Design review of the part built by this model. Coordinates are the model's own, in mm. A direction names the side the tool comes from. Coordinates: 2 decimals unless noted, no trailing zeros. Loops run counter-clockwise (first coordinate to the right, second up) from the corner with the lowest first, then second, coordinate; pieces in that order, holes last.
Q1. For P1, Ø0.6, axis at y = 4.5, z = 0.5, coming from the +X side; P2, Ø0.6, axis at x = -17, z = 1, coming from the -Y side, all flat-tipped, find the tip position at first contact; note any pin that passes through.
Q2. Draft analysis for pull direction Y (two halves, no side actions). For faces 6 (the face through (0.3, 10.305, -0.5)), 7 (the face through (0.252, 4.38, 0.914)), 8 (the face through (0, 14, -1.024)), state which applies: released by +Y, released by -Y, zero draft, split by the parting line, or undercut.
Q3. Add section C-C on y = 4.25. Give the boundary of the cut face in (x, z), and give its area (3 significant figures).
Q4. Machinability: for faces 1 (the face through (0, 8, -0.024)), 2 (the face through (-16, 4, 0.4)), 3 (the face through (16, 4, 0.4)), 4 (the face through (-18, 13, 0)), 5 (the face through (-17.715, 18.003, 0.256)), which of the approach directions +Z, -Z, +X, -X, +Y, -Y give a long, thin tool a straight path to every point of the face, cutting with its end or side? Answer none if there is none.
Q5. Add section A-A on x = 0. Give the boundary of the cut face in (y, z), and give its area (3 significant figures).
Q6. Wall thickness on probe 1 along Y at (x, z) = (-13, -0.55); probe 2 along Z at (x, y) = (-8, 7.25); probe 3 along Z at (x, y) = (-5, 4.5): over which ranges is each line inside the solid? List them lowest first.
Q7. Add section B-B on y = 8.25. Give the boundary of the cut face in (x, z).
```python
from build123d import *

# Parameters (mm, degrees)
BOSS_EXTRUDE1_DEPTH      = 1.5
BOSS_EXTRUDE1_DEPTH_BACK = 1.2
CUT_EXTRUDE1_DEPTH       = 40


with BuildPart() as part:
    # Sketch1 → Boss-Extrude1 (new body, two sides)
    with BuildSketch(Plane.XY) as boss_extrude1_sk:
        with BuildLine():
            Line((-17.999999991, 9.304537824), (-17.999999991, 10.304506021))
            Line((-17.999999991, 10.304506021), (-17.999999991, 17.303464443))
            ThreePointArc((-17.999999991, 17.303464443), (-17.707106772, 18.010571225), (-16.999999991, 18.303464443))
            Line((-16.999999991, 18.303464443), (16.999968161, 18.303464443))
            ThreePointArc((16.999968161, 18.303464443), (17.707074942, 18.010571225), (17.999968161, 17.303464443))
            Line((17.999968161, 17.303464443), (17.999968161, 9.303464443))
            Line((17.999968161, 9.303464443), (17.999968161, 6.751174458))
            ThreePointArc((17.999968161, 6.751174458), (17.707074942, 6.044067677), (16.999968161, 5.751174458))
            Line((16.999968161, 5.751174458), (16.499999991, 5.751174458))
            ThreePointArc((16.499999991, 5.751174458), (16.1464466, 5.604727849), (15.999999991, 5.251174458))
            Line((15.999999991, 5.251174458), (15.999999991, 2.751174458))
            ThreePointArc((15.999999991, 2.751174458), (15.707106772, 2.044067677), (14.999999991, 1.751174458))
            Line((14.999999991, 1.751174458), (-14.999999991, 1.751174458))
            ThreePointArc((-14.999999991, 1.751174458), (-15.707106772, 2.044067677), (-15.999999991, 2.751174458))
            Line((-15.999999991, 2.751174458), (-15.999999991, 5.251174458))
            ThreePointArc((-15.999999991, 5.251174458), (-16.1464466, 5.604727849), (-16.499999991, 5.751174458))
            Line((-16.499999991, 5.751174458), (-16.999999991, 5.751174458))
            ThreePointArc((-16.999999991, 5.751174458), (-17.707106772, 6.044067677), (-17.999999991, 6.751174458))
            Line((-17.999999991, 6.751174458), (-17.999999991, 9.304537824))
        make_face()
    extrude(amount=BOSS_EXTRUDE1_DEPTH)
    extrude(boss_extrude1_sk.sketch, amount=-BOSS_EXTRUDE1_DEPTH_BACK)

    # Sketch3 → Cut-Extrude1 (cut)
    with BuildSketch(Plane(origin=(17.999968161, 0, 0), x_dir=(0, 0, -1), z_dir=(1, 0, 0))):
        with BuildLine():
            Line((0.023796664, 6.751174458), (0.023796664, 5.754537824))
            ThreePointArc((0.023796664, 5.754537824), (0.053060483, 3.748723952), (0.23729316, 1.751174458))
            Line((0.23729316, 1.751174458), (1.2708887, 1.751174458))
            Line((1.2708887, 1.751174458), (1.2708887, 10.304537824))
            Line((1.2708887, 10.304537824), (1.2708887, 10.30507849))
            ThreePointArc((1.2708887, 10.30507849), (7.212872074, 16.614024598), (1.023796664, 22.680762846))
            Line((1.023796664, 22.680762846), (1.023796664, 17.303464443))
            Line((1.023796664, 17.303464443), (1.2, 17.303464443))
            Line((1.2, 17.303464443), (1.2, 6.751174458))
            Line((1.2, 6.751174458), (0.023796664, 6.751174458))
        make_face()
        Polygon((0.023796664, 10.304537824), (0.023796664, 6.751174458), (1.2, 6.751174458), (1.2, 17.303464443), (1.023796664, 17.303464443), (1.023796664, 10.304537824), align=None)
        with BuildLine():
            ThreePointArc((-1.485404738, 6.692099607), (-1.491731963, 6.721473521), (-1.496283327, 6.751174458))
            Line((-1.496283327, 6.751174458), (-1.5, 6.751174458))
            Line((-1.5, 6.751174458), (-1.5, 1.751174458))
            Line((-1.5, 1.751174458), (0.126821568, 1.751174458))
            ThreePointArc((0.126821568, 1.751174458), (-0.181429151, 1.857497567), (-0.358583171, 2.131248481))
            Line((-0.358583171, 2.131248481), (-1.485404738, 6.692099607))
        make_face()
        with BuildLine():
            Line((-1.5, 6.751174458), (-1.496283327, 6.751174458))
            ThreePointArc((-1.496283327, 6.751174458), (-1.499069967, 6.781543322), (-1.5, 6.812025585))
            Line((-1.5, 6.812025585), (-1.5, 6.751174458))
        make_face()
    extrude(amount=-CUT_EXTRUDE1_DEPTH, mode=Mode.SUBTRACT)


solid = part.part
```
Entries:
1. P1: stops at x = 16
1. P2: stops at y = 5.75
2. face 6: undercut
2. face 7: released by -Y
2. face 8: zero draft
3. outline: (-16, -0.03) - (16, -0.03) - (16, 0.88) - (-16, 0.88) - close
3. area: 29.2 mm2
4. face 1: -Z, +X, -X
4. face 2: +Z, -Z, -X, -Y
4. face 3: +Z, -Z, +X, -Y
4. face 4: +Z, -Z, -X, +Y, -Y
4. face 5: +Z, -Z, -X, +Y
5. outline: (1.75, -0.24) arc R25.93 cw to (5.75, -0.02) - (10.3, -0.02) - (10.3, -1.02) - (18.3, -1.02) - (18.3, 1.5) - (6.81, 1.5) arc R0.5 ccw to (6.69, 1.49) - (2.13, 0.36) arc R0.5 ccw to (1.75, -0.13) - close
5. area: 30.3 mm2
6. probe 1: y = 10.3 to 18.3
6. probe 2: z = -0.02 to 1.5
6. probe 3: z = -0.02 to 0.94
7. outline: (-18, -0.02) - (18, -0.02) - (18, 1.5) - (-18, 1.5) - close
